Input: part model. Units: mm. Frame: model coordinates. Give positions to 0.01 mm unless a question says otherwise; leave off trailing zeros. Loops run counter-clockwise (first coordinate to the right, second up) from the corner with the lowest first, then second, coordinate; pieces in that order, holes last. Notation, with made-up numbers: M -25.5,-20.75 L -8.5,-20.75 A31 ccw -8.5,3.25 Z; hole C 42.5,29.25 d5. An arc over 180 degrees is marked long. Answer as a JSON object with one key per item and string values. Group by question number.
```python
from build123d import *

# Parameters (mm, degrees)
SHAFT_BOSS_DEPTH                = 914.4
SKETCH2_R                       = 9.41705
SKETCH2_R_2                     = 6.87705
CUT_FOR_THUNDER_HEX_ROUND_DEPTH = 914.4
SKETCH3_R                       = 2.5527
CENTER_HOLE_CUT_DEPTH           = 914.4


with BuildPart() as part:
    # Sketch1 → Shaft Boss (new body)
    with BuildSketch(Plane.XY):
        Polygon((0, 7.332348419), (-6.35, 3.666174209), (-6.35, -3.666174209), (0, -7.332348419), (6.35, -3.666174209), (6.35, 3.666174209), align=None)
    extrude(amount=SHAFT_BOSS_DEPTH)

    # Sketch2 → Cut For Thunder Hex Round (cut)
    with BuildSketch(Plane(origin=(0, 0, 0), x_dir=(-1, 0, 0), z_dir=(0, 0, -1))):
        Circle(SKETCH2_R)
        Circle(SKETCH2_R_2, mode=Mode.SUBTRACT)
    extrude(amount=-CUT_FOR_THUNDER_HEX_ROUND_DEPTH, mode=Mode.SUBTRACT)

    # Sketch3 → Center Hole Cut (cut)
    with BuildSketch(Plane(origin=(0, 0, 0), x_dir=(-1, 0, 0), z_dir=(0, 0, -1))):
        Circle(SKETCH3_R)
    extrude(amount=-CENTER_HOLE_CUT_DEPTH, mode=Mode.SUBTRACT)


solid = part.part
```
1. Section B-B (z = 347). Output: boundary loops of the cut face in (x, y).
2. First-contact query: P1, Ø2, axis at y = 4, z = 232.5, coming from the -X side; P2, Ø1, axis at x = 2.5, z = 106.5, coming from the +Y side; P3, Ø5, axis at x = 3, z = 724.5, coming from the +Y side. Flat tips, straight axial feed; report the tip coordinate or a pass-through.
3. Section A-A (y = 0). Output: boundary loops of the cut face in (x, z).
4. Material intervals for L1, parallel to Y at x = 0, z = 728.5; L2, parallel to Y at x = 0.25, z = 552; L3, parallel to X at y = -0.5, z = 767, sorted ascending.
Geometry results:
{
 "1": {"outline": "M -6.35,-2.64 A6.88 ccw -5.46,-4.18 L -0.89,-6.82 A6.88 ccw 0.89,-6.82 L 5.46,-4.18 A6.88 ccw 6.35,-2.64 L 6.35,2.64 A6.88 ccw 5.46,4.18 L 0.89,6.82 A6.88 ccw -0.89,6.82 L -5.46,4.18 A6.88 ccw -6.35,2.64 Z; hole C 0,0 d5.11"},
 "2": {"P1": "x = -6.19", "P2": "y = 6.18", "P3": "y = 6.86"},
 "3": {"outline": "M -6.35,0 L -2.55,0 L -2.55,914.4 L -6.35,914.4 Z; M 2.55,0 L 6.35,0 L 6.35,914.4 L 2.55,914.4 Z"},
 "4": {"L1": "-6.88 to -2.55, 2.55 to 6.88", "L2": "-6.87 to -2.54, 2.54 to 6.87", "L3": "-6.35 to -2.5, 2.5 to 6.35"}
}
